Geometry check sheet. Reference: the model listing, model coordinates, mm. A direction names the side the tool comes from. Coordinates: 2 decimals unless noted, no trailing zeros. Write each loop counter-clockwise with the first axis right and the second up, starting at its lowest first coordinate (ties: lowest second). Pieces come first, ordered by that corner, then holes. Notation, with made-up numbers: (-7, -9) -> (-3, -9) arc R19 ccw to (-3, -2) -> close; hole circle Ø11 at (20, 9). An arc over 180 degrees is marked (long way). Answer in a Markdown table with one row per item. Add a question column.
1. Mould release check, pull along X, two halves, no side actions. Record for faces 1 (the cylindrical face through (0.217, -3.377, -0.004)), 2 (the flat face through (0, 5, 3)), 3 (the flat face through (-2, 4, 1)): pulls with the +X half, pulls with the -X half, needs draft (parallel to the pull), parting line crosses it, or undercut.
2. Cross-section at D-D on y = 4.5. Record the cut outline in (x, z).
3. Set-up check for faces 4 (the flat face through (0, 4.1, 0.3)), 5 (the flat face through (0, -1, -0.25)), 6 (the flat face through (0, 1, 0.5)): record each of +Z, -Z, +X, -X, +Y, -Y from which the full face is reachable in a straight line by a thin tool's end or side.
4. Scan lines: L1, parallel to Y at x = -0.95, z = 4.25; L2, parallel to Z at x = 0, y = 0.75; L3, parallel to Z at x = 1.65, y = -2. Record each from-to range of solid material in increasing order. Write a range as from..to.
5. Cross-section at C-C on y = -2.25. Record the cut outline in (x, z), and give its area (3 significant figures).
6. Depth check by flat-ended pin: P1, Ø0.6, axis at y = -3, z = 0, coming from the -X side; P2, Ø1, axis at x = 0, y = -2.5, coming from the +Z side; P3, Ø1.5, axis at x = 1.5, z = 2, coming from the -Y side. Enter the tip coordinate at first touch or a pass-through.
```python
from build123d import *

# Parameters (mm, degrees)
SZKIC1_W                    = 4
SZKIC1_H                    = 1
DODANIE_WYCI_GNI_CIE5_DEPTH = 5
SZKIC6_W                    = 4
SZKIC6_H                    = 1
DODANIE_WYCI_GNI_CIE6_DEPTH = 4.5
SFAZOWANIE2_SIZE            = 1
SFAZOWANIE4_SIZE            = 1.7
SZKIC13_W                   = 3.5
SZKIC13_H                   = 0.5
DODANIE_WYCI_GNI_CIE7_DEPTH = 3.9
ZAOKR_GLENIE1_R             = 0.25
SZKIC14_R                   = 1
WYTNIJ_WYCI_GNI_CIE1_DEPTH  = 3.9
ZAOKR_GLENIE2_R             = 0.25


with BuildPart() as part:
    # Szkic1 → Dodanie-wyciągnięcie5 (new body)
    with BuildSketch(Plane(origin=(0, 0, 0), x_dir=(1, 0, 0), z_dir=(0, 1, 0))):
        Rectangle(SZKIC1_W, SZKIC1_H)
    extrude(amount=DODANIE_WYCI_GNI_CIE5_DEPTH)

    # Szkic6 → Dodanie-wyciągnięcie6 (add)
    with BuildSketch(Plane.XY.offset(0.5)):
        with Locations((0, 4.5)):
            Rectangle(SZKIC6_W, SZKIC6_H)
    extrude(amount=DODANIE_WYCI_GNI_CIE6_DEPTH)

    # Sfazowanie2
    sfazowanie2_edges = [part.edges().sort_by_distance(p)[0] for p in [
        (0, 4, 0.5),
    ]]
    chamfer(sfazowanie2_edges, length=SFAZOWANIE2_SIZE)

    # Sfazowanie4
    sfazowanie4_edges = [part.edges().sort_by_distance(p)[0] for p in [
        (0, 5, -0.5),
    ]]
    chamfer(sfazowanie4_edges, length=SFAZOWANIE4_SIZE)

    # Szkic13 → Dodanie-wyciągnięcie7 (add)
    with BuildSketch(Plane.XZ):
        Rectangle(SZKIC13_W, SZKIC13_H)
    extrude(amount=DODANIE_WYCI_GNI_CIE7_DEPTH)

    # Zaokrąglenie1
    zaokr_glenie1_edges = [part.edges().sort_by_distance(p)[0] for p in [
        (-1.75, 0, 0),
        (0, 0, -0.25),
        (1.75, 0, 0),
        (0, 0, 0.25),
    ]]
    fillet(zaokr_glenie1_edges, radius=ZAOKR_GLENIE1_R - 0.0001)  # a hair under: the kernel refuses the full size

    # Szkic14 → Wytnij-wyciągnięcie1 (cut)
    with BuildSketch(Plane(origin=(0, 0, -0.25), x_dir=(-1, 0, 0), z_dir=(0, 0, -1))):
        with Locations((0, -2.400763045)):
            Circle(SZKIC14_R)
    extrude(amount=-WYTNIJ_WYCI_GNI_CIE1_DEPTH, mode=Mode.SUBTRACT)

    # Zaokrąglenie2
    zaokr_glenie2_edges = [part.edges().sort_by_distance(p)[0] for p in [
        (-1.75, -3.9, 0),
        (1.75, -3.9, 0),
    ]]
    fillet(zaokr_glenie2_edges, radius=ZAOKR_GLENIE2_R)


solid = part.part
```
Results found:
| question | item | result |
|---|---|---|
| 1 | face 1 | undercut |
| 1 | face 2 | needs draft |
| 1 | face 3 | pulls with the -X half |
| 2 | outline | (-2, 0.7) -> (2, 0.7) -> (2, 5) -> (-2, 5) -> close |
| 3 | face 4 | -Z, +X, -X, +Y |
| 3 | face 5 | -Z, +X, -X, -Y |
| 3 | face 6 | +Z, +X, -X, -Y |
| 4 | L1 | y = 4..5 |
| 4 | L2 | z = -0.5..0.5 |
| 4 | L3 | z = -0.25..0.25 |
| 5 | outline | (-1.75, -0.25) -> (-0.99, -0.25) -> (-0.99, 0.25) -> (-1.75, 0.25) -> close; (0.99, -0.25) -> (1.75, -0.25) -> (1.75, 0.25) -> (0.99, 0.25) -> close |
| 5 | area | 0.761 mm^2 |
| 6 | P1 | stops at x = -1.75 |
| 6 | P2 | passes through |
| 6 | P3 | stops at y = 3.75 |
